Could you check a few things on this model? Use its own coordinates, in mm. A direction names the side the tool comes from. Coordinates: 2 decimals unless noted, no trailing zeros. Write each loop counter-clockwise with the first axis right and the second up, starting at its lowest first coordinate (ties: lowest second). Pieces come first, ordered by that corner, then holes. Notation, with made-up numbers: M 49,-23 L 93,-23 A15 cw 93,5 Z; hole C -35.75,-15.5 d6. An arc over 180 degrees is marked long. Answer as CSV lines item,"result". Start each with the question number.
Item 1: On a 3-axis mill with a long thin cutter (end or side, diameter ignored), from which of +Z, -Z, +X, -X, +Y, -Y can I reach the whole of each face in a straight line? I mean faces 1 (the cylindrical face through (2.5, 3.94, -1.43)), 2 (the flat face through (1, -1.5, -1)). Say none if no direction works.
Item 2: Suppose I cut it at A-A, the plane x = 0. Write out the boundary of the cut face in (y, z).
Item 3: Suppose I cut it at B-B, the plane z = 0. Write out the boundary of the cut face in (x, y).
Item 4: We'd pull the mould along X, two halves only. Please class faces 3 (the cylindrical face through (-0.976, -0.74, 4.397)), 4 (the cylindrical face through (0.01, 3.94, -2.88)), 5 (the flat face through (-2, 8, 0)): +X half, -X half, draft (parallel to the pull), parting line (faces both ways), or undercut.
Item 5: If I drill on line 1 along X through (y, z) = (3, 0); line 2 along Z through (x, y) = (0, -0.7), over which ranges is the centre line in solid material (lowest first)? Write a range as [from, to].
Item 6: I'm going to push flat-ended pins straight in: P1, Ø2, axis at x = 2, y = 6, coming from the +Z side; P2, Ø2, axis at y = 6, z = -1.5, coming from the -X side; P3, Ø1.5, axis at y = 5.5, z = 2.5, coming from the -X side. Where does each tip first touch, or does it pass through?
Item 7: Suppose I cut it at C-C, the plane x = 3.75. Write out the boundary of the cut face in (y, z).
Autodesk Inventor part; units mm, degrees
ref_plane "YZ Plane" through (0, 0, 0) normal (1, 0, 0) x (0, 1, 0)
ref_plane "XZ Plane" through (0, 0, 0) normal (0, 1, 0) x (-1, 0, 0)
ref_plane "XY Plane" through (0, 0, 0) normal (0, 0, 1) x (1, 0, 0)
sketch "Sketch1" plane through (0, 0, 0) normal (0, 1, 0) x (-1, 0, 0)
  circle A0 centre (0, 0) radius 1.2
  circle A1 centre (0, 0) radius 3.6287
  dimension "BoreD" = 2.4
  dimension "OuterD" = 7.2575
extrude "Extrusion1" add sketch "Sketch1" along normal blind 8
sketch "Sketch2" plane through (0, 0, 0) normal (0, -1, 0) x (1, 0, 0)
  circle A0 centre (0, 0) radius 3.6287
  arc A1 (0.4991, -3.4087) -> (0.6768, -3.5651) centre (0.6488, -3.4177) ccw
  arc A2 (0.4991, -3.4087) -> (-0.4991, -3.4087) centre (0, -3.3787) ccw
  arc A3 (-0.6768, -3.5651) -> (-0.4991, -3.4087) centre (-0.6488, -3.4177) ccw
  point P0 (0, -3.6287)
  dimension "d9" = 0.5
  dimension "d10" = 0.15
  dimension "Depth" = 0.25
extrude "Extrusion2" cut sketch "Sketch2" against normal up to next contours A3 A2 A1 A0 picked at (0, -3.374)
pattern_circular "Circular Pattern1" count 12 over 360 about axis through (0, -10, 0) along (0, 1, 0) of "Extrusion2"
sketch "Sketch3" plane through (0, 0, 0) normal (0, -1, 0) x (1, 0, 0)
  circle A0 centre (0, 0) radius 4.5037
  circle A1 centre (0, 0) radius 1.2
  dimension "FaceD" = 9.0075
  dimension "d18" = 2.4
extrude "Extrusion3" add sketch "Sketch3" along normal blind 1.5
equation "\"OuterD\" = 0.0604789 * Teeth"
equation "\"d18\" = BoreD"
equation "\"BeltWidth\" = 7"
equation "\"Pitch\" = 0.25"
properties part number "GT2 Gear Pinion"
Ans:
1,face 1,"+Y"
1,face 2,"+Z, -Z, +X, -X, -Y"
2,outline,"M -1.5,-4.5 L 0,-4.5 L 0,-2.88 L 8,-2.88 L 8,-1.2 L -1.5,-1.2 Z; M -1.5,1.2 L 8,1.2 L 8,2.88 L 0,2.88 L 0,4.5 L -1.5,4.5 Z"
3,outline,"M -4.5,-1.5 L -1.2,-1.5 L -1.2,8 L -2.88,8 L -2.88,0 L -4.5,0 Z; M 1.2,-1.5 L 4.5,-1.5 L 4.5,0 L 2.88,0 L 2.88,8 L 1.2,8 Z"
4,face 3,"parting line"
4,face 4,"undercut"
4,face 5,"draft"
5,line 1,"x = [-2.88, -1.2], [1.2, 2.88]"
5,line 2,"z = [-4.5, -1.2], [1.2, 4.5]"
6,P1,"stops at z = 3.49"
6,P2,"stops at x = -3.57"
6,P3,"stops at x = -2.79"
7,outline,"M -1.5,-2.49 L 0,-2.49 L 0,2.49 L -1.5,2.49 Z"
